Model file for the job. Use its own axes, mm. A direction names the side the tool comes from. Round coordinates to 2 decimals unless told otherwise and drop trailing zeros. Loops run counter-clockwise (first coordinate to the right, second up) from the corner with the lowest first, then second, coordinate; pieces in that order, holes last. Notation, with made-up numbers: M -7.5,87.5 L 1.5,87.5 A36 ccw 1.5,123.5 Z; hole C 86,57 d1. An arc over 180 degrees is marked long. Use a Markdown table: item, result. Add a question column.
Item 1: Saw through at C-C on y = 6.5. Write the cut outline in (x, z) (1 decimal).
Item 2: Saw through at B-B on x = 31.75. Write the cut outline in (y, z), then the cut area to 3 significant figures.
Item 3: Saw through at A-A on z = 19.05. Give the number of separate pieces and of enclosed holes in the cut face, then the cut area to 3 significant figures.
Item 4: Saw through at D-D on z = -36.5. Write the cut outline in (x, y).
Item 5: Pin check, flat tips, straight feed: P1, Ø5, axis at y = 29.5, z = -32, coming from the +X side; P2, Ø11.5, axis at x = 41, z = 15.5, coming from the +Y side; P3, Ø6, axis at x = 16, y = 11, coming from the -Z side; P4, Ø3, axis at x = 16.5, z = -5.5, coming from the +Y side. Stop position of each tip, or through.
Item 6: Tool access for faces 1 (the flat face through (74.243, 28.361, -23.23)), 2 (the cylindrical face through (26.92, -3.91, 12.75)), 3 (the flat face through (9.525, 11, 10)), 4 (the flat face through (36.621, 45.435, -19.544)): list every direction of +Z, -Z, +X, -X, +Y, -Y with a clear straight run to the whole face (end or side of a thin tool).
Item 7: Two-plate mould, pull along X, no slides. Class faces 5 (the flat face through (36, 28, 0)), 6 (the cylindrical face through (63.79, 34.4, -29.06)), 7 (the flat face through (1.96, 69.97, -18.78)): +X half, -X half, draft (parallel to the pull), parting line (faces both ways), or undercut.
Item 8: Wall check: L1, parallel to X at y = -4, z = 19.05; L2, parallel to Z at x = 27, y = 55.5; L3, parallel to Y at x = 23, z = 30. Give the ranges that are in metal, low to high. Write a range as from..to.
```python
from build123d import *

# Parameters (mm, degrees)
BASE_EXTRUDE_THIN_DEPTH = 76.2
BOSS_EXTRUDE1_START     = -7.9375
BOSS_EXTRUDE1_DEPTH     = 7.9375
SKETCH3_W               = 87.988181024
SKETCH3_H               = 50.8
BOSS_EXTRUDE2_DEPTH     = 7.9375
CUT_EXTRUDE1_DEPTH      = 119.845476344
FILLET1_R               = 12.7
BOSS_EXTRUDE3_DEPTH     = 9.525
CUT_EXTRUDE2_DEPTH      = 100.992371073
SKETCH9_R               = 7.9375
CUT_EXTRUDE3_DEPTH      = 118.398397707
LPATTERN2_COUNT         = 2
LPATTERN2_PITCH         = 28.575


# Read off the part's stored shape, not the designer's step: Boss-Extrude1
with BuildPart() as part:
    # Sketch1 → Base-Extrude-Thin (new body)
    with BuildSketch(Plane(origin=(0, 0, 0), x_dir=(0, 0, -1), z_dir=(1, 0, 0))):
        Polygon((-38.1, 0), (0, 0), (0, 31.75), (7.9375, 31.75), (7.9375, -7.9375), (-38.1, -7.9375), align=None)
    extrude(amount=BASE_EXTRUDE_THIN_DEPTH)

    # Boss-Extrude1 outline → Boss-Extrude1 (add)
    with BuildSketch(Plane.XY.offset(BOSS_EXTRUDE1_START)):
        Polygon((76.2, 31.75), (0, 75.744090512), (0, 31.75), align=None)
    extrude(amount=BOSS_EXTRUDE1_DEPTH)

    # Sketch3 → Boss-Extrude2 (add)
    with BuildSketch(Plane(origin=(32.798153285, 56.808067884, 0), x_dir=(-0.8660254037844379, 0.5000000000000014, 0), z_dir=(0.5000000000000014, 0.8660254037844379, 0))):
        with Locations((-6.122045256, -25.4)):
            Rectangle(SKETCH3_W, SKETCH3_H)
    extrude(amount=-BOSS_EXTRUDE2_DEPTH)

    # Sketch4 → Cut-Extrude1 (cut, through all)
    with BuildSketch(Plane.XY):
        Polygon((-113.819682418, -130.562817861), (0, 66.578654989), (3.96875, 73.452731631), (117.788432418, 270.594204481), (-276.494513281, 498.233569317), (-508.102628117, 97.076546976), align=None)
    extrude(amount=-CUT_EXTRUDE1_DEPTH, mode=Mode.SUBTRACT)

    # Fillet1
    fillet1_edges = [part.edges().sort_by_distance(p)[0] for p in [
        (74.215625, 28.312961679, -50.8),
        (1.984375, 70.01569331, -50.8),
    ]]
    fillet(fillet1_edges, radius=FILLET1_R)

    # Sketch5 → Boss-Extrude3 (add)
    with BuildSketch(Plane.ZY):
        Polygon((0, 38.1), (0, 0), (38.1, 0), align=None)
    extrude(amount=-BOSS_EXTRUDE3_DEPTH)

    # Sketch6 → Cut-Extrude2 (cut, through all)
    with BuildSketch(Plane(origin=(24.654916237, 61.509567986, -0.61351416), x_dir=(-0.866025403784438, 0.5000000000000012, 0), z_dir=(0.5000000000000011, 0.8660254037844379, 0))):
        with BuildLine():
            Line((-0.781635971, -34.70836084), (-22.616879552, -34.70836084))
            ThreePointArc((-22.616879552, -34.70836084), (-47.454135971, -27.96148584), (-22.616879552, -21.21461084))
            Line((-22.616879552, -21.21461084), (-0.781635971, -21.21461084))
            ThreePointArc((-0.781635971, -21.21461084), (5.965239029, -27.96148584), (-0.781635971, -34.70836084))
        make_face()
    extrude(amount=-CUT_EXTRUDE2_DEPTH, mode=Mode.SUBTRACT)

    # Sketch9 → Cut-Extrude3 (cut, through all)
    with BuildSketch(Plane(origin=(0, 0, 0), x_dir=(-1, 0, 0), z_dir=(0, 1, 0))):
        with Locations(Location((-60.325, 19.05, 0), (0, 0, 90))):
            Circle(SKETCH9_R)
    cut_extrude3 = extrude(amount=-CUT_EXTRUDE3_DEPTH, mode=Mode.SUBTRACT)

    # LPattern2: Cut-Extrude3 ×2
    with Locations(*[(-i * LPATTERN2_PITCH, 0, 0) for i in range(1, LPATTERN2_COUNT)]):
        add(cut_extrude3, mode=Mode.SUBTRACT)


solid = part.part
```
Entries:
| question | item | result |
|---|---|---|
| 1 | outline | M 0,-7.9 L 76.2,-7.9 L 76.2,0 L 9.5,0 L 9.5,31.6 L 0,31.6 Z |
| 2 | outline | M -7.94,-7.94 L 48.25,-7.94 L 48.25,-21.83 L 57.41,-21.83 L 57.41,0 L 0,0 L 0,11.11 L -7.94,11.11 Z; M -7.94,26.99 L 0,26.99 L 0,38.1 L -7.94,38.1 Z; M 48.25,-50.8 L 57.41,-50.8 L 57.41,-35.32 L 48.25,-35.32 Z |
| 2 | area | 964 mm2 |
| 3 | separate pieces | 3 |
| 3 | enclosed holes | 0 |
| 3 | area | 534 mm2 |
| 4 | outline | M 0,66.58 L 40.95,42.94 L 44.92,49.81 L 3.97,73.45 Z; M 59.52,32.21 L 72.23,24.88 L 76.2,31.75 L 63.49,39.09 Z |
| 5 | P1 | x = 76.2 |
| 5 | P2 | y = 0 |
| 5 | P3 | z = -7.94 |
| 5 | P4 | y = 67.08 |
| 6 | face 1 | -Z, +X, -Y |
| 6 | face 2 | +Y, -Y |
| 6 | face 3 | +Z, +X, +Y |
| 6 | face 4 | -Z, -X, -Y |
| 7 | face 5 | draft |
| 7 | face 6 | undercut |
| 7 | face 7 | -X half |
| 8 | L1 | 0..23.81, 39.69..52.39, 68.26..76.2 |
| 8 | L2 | -50.8..-35.32, -21.83..0 |
| 8 | L3 | -7.94..0 |
